The drawing under review shows one solid part. Ordinate dimensions are in mm from its lowest x, y, z. A direction names the side the tool comes from. Round coordinates to 2 decimals unless told otherwise and drop trailing zeros. Write each loop counter-clockwise with the first axis right and the second up, starting at its lowest first coordinate (ties: lowest second). Pieces come first, ordered by that corner, then holes. Notation, with made-up numbers: (84.5, 0) -> (134.5, 0) arc R7 ccw to (134.5, 6) -> close; hole circle Ø2 at (87.5, 83.25). An arc over 180 degrees is marked (long way). Write item = value, one per line. Start each with the question number.
Item 1: Add section B-B, the plane x = 28. State the section outline as (y, z) points, then the cut area to 3 significant figures.
Item 2: Add section D-D, the plane y = 6. State the section outline as (x, z) points, then the cut area to 3 significant figures.
Item 3: Add section C-C, the plane x = 10.5. State the section outline as (y, z) points, then the cut area to 3 significant figures.
Item 4: To check wall thickness, follow L1, parallel to X at y = 22, z = 63; L2, parallel to X at y = 21, z = 63.5; L3, parallel to Z at x = 6.5, y = 18.5. State the ranges of each line that lie inside material, in increasing order.
Item 5: Mouldability with a two-part tool opening along Z and no side actions: class the marked faces 1, 2 and 3 as released by +Z, released by -Z, zero draft, split by the parting line, or undercut.
Item 6: Add section A-A, the plane z = 63.5. State the section outline as (x, y) points, then the cut area to 3 significant figures.
Item 7: Machinability: for the marked faces 4 and 5, which of the approach directions +Z, -Z, +X, -X, +Y, -Y give a long, thin tool a straight path to every point of the face, cutting with its end or side? Answer none if there is none.
Item 8: For pin 1 Ø8 at (x, z) = (24, 30.5) entering from -Y; pin 2 Ø4 at (x, y) = (35, 5) entering from -Z; pin 3 Ø12.5 at (x, z) = (24, 143) entering from -Y, all flat-tipped, find the tip position at first contact; note any pin that passes through.
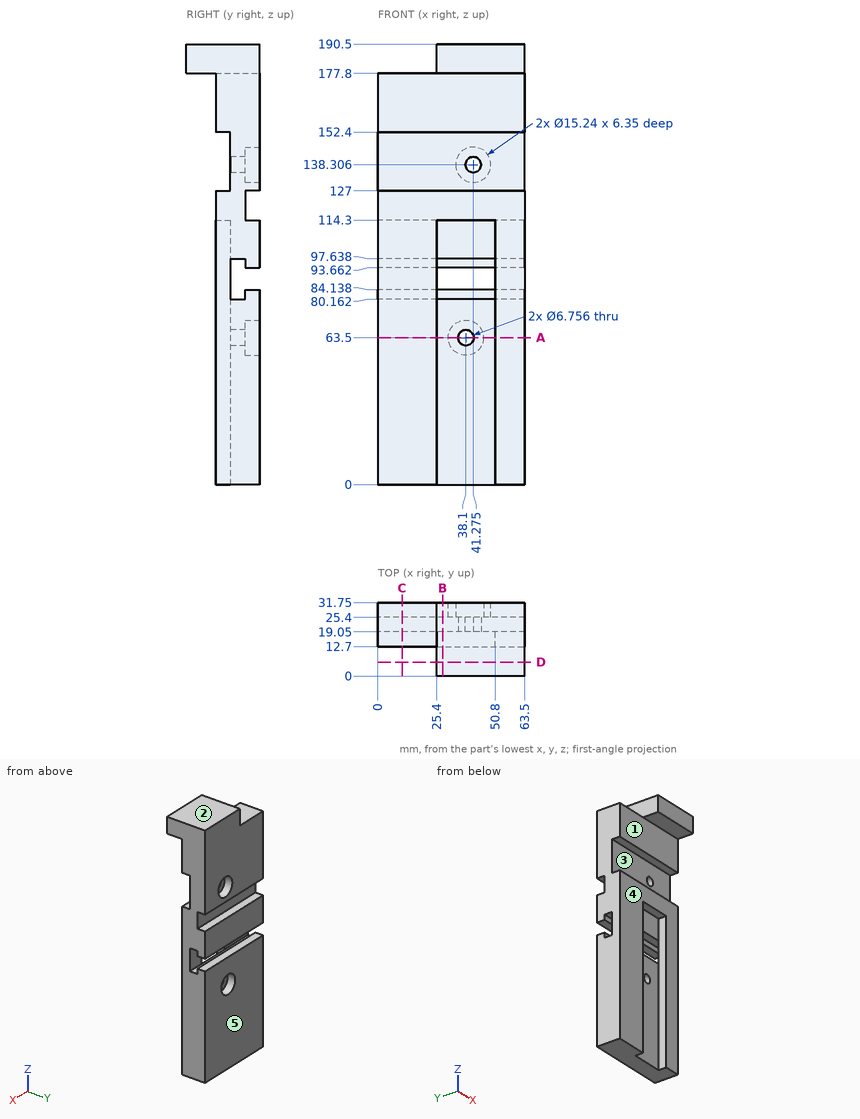
Result set:
q1.outline = (0, 177.8) -> (12.7, 177.8) -> (12.7, 152.4) -> (19.05, 152.4) -> (19.05, 127) -> (12.7, 127) -> (12.7, 114.3) -> (19.05, 114.3) -> (19.05, 97.64) -> (25.4, 97.64) -> (25.4, 93.66) -> (31.75, 93.66) -> (31.75, 114.3) -> (25.4, 114.3) -> (25.4, 127) -> (31.75, 127) -> (31.75, 190.5) -> (0, 190.5) -> close; (19.05, 0) -> (31.75, 0) -> (31.75, 84.14) -> (25.4, 84.14) -> (25.4, 80.16) -> (19.05, 80.16) -> close
q1.area = 2,650 mm²
q2.outline = (25.4, 177.8) -> (63.5, 177.8) -> (63.5, 190.5) -> (25.4, 190.5) -> close
q2.area = 484 mm²
q3.outline = (12.7, 0) -> (31.75, 0) -> (31.75, 84.14) -> (25.4, 84.14) -> (25.4, 80.16) -> (19.05, 80.16) -> (19.05, 97.64) -> (25.4, 97.64) -> (25.4, 93.66) -> (31.75, 93.66) -> (31.75, 114.3) -> (25.4, 114.3) -> (25.4, 127) -> (31.75, 127) -> (31.75, 177.8) -> (12.7, 177.8) -> (12.7, 152.4) -> (19.05, 152.4) -> (19.05, 127) -> (12.7, 127) -> close
q3.area = 2,970 mm²
q4.L1 = 0 to 34.76, 41.44 to 63.5
q4.L2 = 0 to 34.72, 41.48 to 63.5
q4.L3 = 0 to 127, 152.4 to 177.8
q5.face_1 = zero draft
q5.face_2 = released by +Z
q5.face_3 = undercut
q6.outline = (0, 12.7) -> (25.4, 12.7) -> (25.4, 19.05) -> (34.72, 19.05) -> (34.72, 25.4) -> (30.48, 25.4) -> (30.48, 31.75) -> (0, 31.75) -> close; (41.48, 19.05) -> (50.8, 19.05) -> (50.8, 12.7) -> (63.5, 12.7) -> (63.5, 31.75) -> (45.72, 31.75) -> (45.72, 25.4) -> (41.48, 25.4) -> close
q6.area = 909 mm²
q7.face_4 = -Z, +X, -X, -Y
q7.face_5 = +Z, -Z, +X, -X, +Y
q8.pin_1 = 12.7
q8.pin_2 = 177.8
q8.pin_3 = 19.05
